from build123d import *

# Parameters (mm, degrees)
BOSS_EXTRUDE1_DEPTH = 393.7
FILLET1_R           = 1.5875


with BuildPart() as part:
    # Sketch1 → Boss-Extrude1 (new body, symmetric)
    with BuildSketch(Plane(origin=(0, 0, 0), x_dir=(0, 0, -1), z_dir=(1, 0, 0))):
        with BuildLine():
            Line((-1.5875, 28.575), (-7.9375, 28.575))
            Line((-7.9375, 28.575), (-7.9375, -1.5875))
            ThreePointArc((-7.9375, -1.5875), (0, -9.525), (7.9375, -1.5875))
            Line((7.9375, -1.5875), (7.9375, 28.575))
            Line((7.9375, 28.575), (1.5875, 28.575))
            Line((1.5875, 28.575), (1.5875, 0))
            Line((1.5875, 0), (-1.5875, 0))
            Line((-1.5875, 0), (-1.5875, 28.575))
        make_face()
    extrude(amount=BOSS_EXTRUDE1_DEPTH, both=True)

    # Fillet1
    fillet1_edges = [part.edges().sort_by_distance(p)[0] for p in [
        (0, 28.575, -7.9375),
        (0, 28.575, 7.9375),
    ]]
    fillet(fillet1_edges, radius=FILLET1_R)


solid = part.part
The model under review builds one solid part; all positions refer to its coordinate system, in mm. Give positions to 0.01 mm unless a question says otherwise; leave off trailing zeros. Write each loop counter-clockwise with the first axis right and the second up, starting at its lowest first coordinate (ties: lowest second). Pieces come first, ordered by that corner, then holes.
1. For P1, Ø1, axis at x = 210, z = -5, coming from the -Y side; P2, Ø1, axis at x = 117.5, z = -0.5, coming from the +Y side; P3, Ø1.5, axis at x = -233.5, z = -6, coming from the -Y side, all flat-tipped, find the tip position at first contact; note any pin that passes through.
2. Add section A-A, the plane y = 7. Write out the cut boundary in (x, z), plus the area to 4 significant figures.
3. Draft analysis for pull direction Z (two halves, no side actions). For faces 1 (the cylindrical face through (5.512, -9.523, 0.175)), 2 (the flat face through (6, 14, -1.588)), 3 (the flat face through (6, 14, 1.588)), 4 (the flat face through (-393.7, 10, -2)), state which applies: +Z half, -Z half, draft (parallel to the pull), parting line (faces both ways), or undercut.
4. Wall thickness on L1, parallel to Z at x = 34, y = 21.5; L2, parallel to Y at x = 23, z = -0.5; L3, parallel to Y at x = -220.5, z = -4.5 (3 decimals): over which ranges is each line inside the solid? List them lowest first.
Worked answers:
1. P1: stops at y = -8.13
1. P2: stops at y = 0
1. P3: stops at y = -7.54
2. outline: (-393.7, -7.94) - (393.7, -7.94) - (393.7, -1.59) - (-393.7, -1.59) - close; (-393.7, 1.59) - (393.7, 1.59) - (393.7, 7.94) - (-393.7, 7.94) - close
2. area: 10,000 mm2
3. face 1: parting line
3. face 2: undercut
3. face 3: undercut
3. face 4: draft
4. L1: z = -7.94 to -1.59, 1.59 to 7.94
4. L2: y = -9.51 to 0
4. L3: y = -8.126 to 28.575
